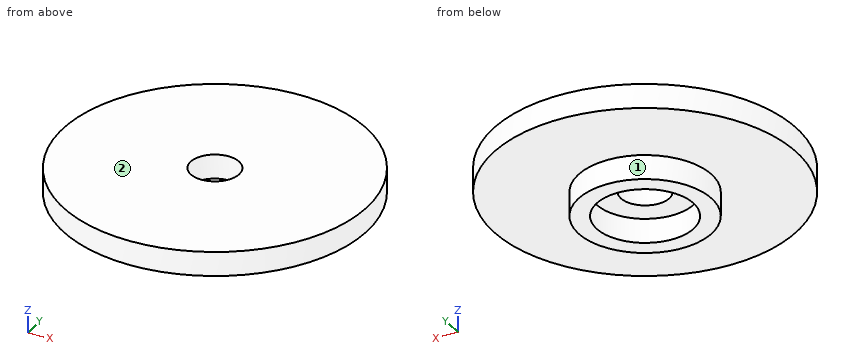
Autodesk Inventor part; units mm, degrees
ref_plane "YZ Plane" through (0, 0, 0) normal (1, 0, 0) x (0, 1, 0)
ref_plane "XZ Plane" through (0, 0, 0) normal (0, 1, 0) x (-1, 0, 0)
ref_plane "XY Plane" through (0, 0, 0) normal (0, 0, 1) x (1, 0, 0)
sketch "Sketch1" plane through (0, 0, 0) normal (0, 0, 1) x (1, 0, 0)
  circle A0 centre (0, 0) radius 12.5
  circle A1 centre (0, 0) radius 4
  circle A2 centre (0, 0) radius 5.5
  dimension "d0" = 25
  dimension "d1" = 8
  dimension "d2" = 11
extrude "Extrusion1" add sketch "Sketch1" against normal blind 2 contours A2
extrude "Extrusion2" add sketch "Sketch1" along normal blind 2 contours A0 | A1 | A2
sketch "Sketch2" plane through (0, 0, 2) normal (0, 0, 1) x (1, 0, 0)
  circle A0 centre (0, 0) radius 2
  dimension "d7" = 4
extrude "Extrusion3" cut sketch "Sketch2" against normal up to next
properties part number "Stepper Cap"
Build history of the part. All positions in model axes, mm. Face numbers are marked on the shaded views. A direction names the side the tool comes from. Coordinates: 2 decimals unless noted, no trailing zeros. Write each loop counter-clockwise with the first axis right and the second up, starting at its lowest first coordinate (ties: lowest second). Pieces come first, ordered by that corner, then holes.
1. 3-axis set-ups, long thin cutter, end or side, ignore diameter. For the marked faces 1 and 2: which of +Z, -Z, +X, -X, +Y, -Y reach the whole face in a straight line?
Answer block:
face 1: -Z
face 2: +Z, +X, -X, +Y, -Y
2. Band-saw the part on C-C, the plane z = 1.6. Give the cut face in (x, y).
Answer block:
outline: circle Ø25 at (0, 0); hole circle Ø4 at (0, 0)
3. Drill centre lines: probe 1 along Y at (x, z) = (0, -0.4); probe 2 along Y at (x, z) = (0, 0.6); probe 3 along Z at (x, y) = (5.5, -0.75). Where is each one in solid material? Low to high.
Answer block:
probe 1: y = -5.5 to -4, 4 to 5.5
probe 2: y = -12.5 to -2, 2 to 12.5
probe 3: z = 0 to 2
4. Band-saw the part on A-A, the plane x = 0. Give the cut face in (y, z).
Answer block:
outline: (-12.5, 0) - (-5.5, 0) - (-5.5, -2) - (-4, -2) - (-4, 0) - (-2, 0) - (-2, 2) - (-12.5, 2) - close; (2, 0) - (4, 0) - (4, -2) - (5.5, -2) - (5.5, 0) - (12.5, 0) - (12.5, 2) - (2, 2) - close
5. Band-saw the part on D-D, the plane y = 3. Give the cut face in (x, z).
Answer block:
outline: (-12.13, 0) - (-4.61, 0) - (-4.61, -2) - (-2.65, -2) - (-2.65, 0) - (2.65, 0) - (2.65, -2) - (4.61, -2) - (4.61, 0) - (12.13, 0) - (12.13, 2) - (-12.13, 2) - close
6. Drop flat-ended pins along their axis: pin 1 (7 mm diameter, centred on x = 0, y = 0, fed in from -Z); pin 2 (1 mm diameter, centred on x = -2.5, z = -1, fed in from +Y). Give the stop position or say it passes through.
Answer block:
pin 1: stops at z = 0
pin 2: stops at y = 5.12
